Build history of the part. All positions in model axes, mm. Face numbers are marked on the shaded views. Coordinates: 2 decimals unless noted, no trailing zeros. Order: outer loops, then holes, each group sorted by start corner. A loop starts at its lowest first (then second) coordinate and runs counter-clockwise, first axis right, second up. Notation, with made-up numbers: (-8, 87) - (26, 87) arc R31 ccw to (26, 112) - close; hole circle Ø1 at (32, -15). An arc over 180 degrees is marked (long way). Write each question's results on one line, items separated by ' | '.
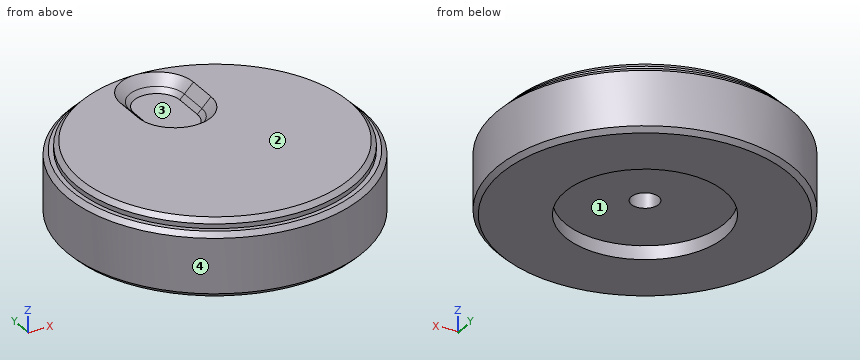
from build123d import *

# Parameters (mm, degrees)
CROQUIS1_R              = 32.5
CROQUIS1_R_2            = 3
SALIENTE_EXTRUIR1_DEPTH = 14
CROQUIS2_R              = 17.5
CORTAR_EXTRUIR1_DEPTH   = 3
CROQUIS3_R              = 30.5
SALIENTE_EXTRUIR2_DEPTH = 2
CHAFL_N1_SIZE           = 1
CORTAR_EXTRUIR2_DEPTH   = 3
CHAFL_N2_SIZE           = 2
SALIENTE_EXTRUIR3_START = 1
SALIENTE_EXTRUIR3_DEPTH = 1
CHAFL_N3_SIZE           = 1


with BuildPart() as part:
    # Croquis1 → Saliente-Extruir1 (new body)
    with BuildSketch(Plane.XY):
        Circle(CROQUIS1_R)
        Circle(CROQUIS1_R_2, mode=Mode.SUBTRACT)
    extrude(amount=SALIENTE_EXTRUIR1_DEPTH)

    # Croquis2 → Cortar-Extruir1 (cut)
    with BuildSketch(Plane(origin=(0, 0, 0), x_dir=(-1, 0, 0), z_dir=(0, 0, -1))):
        Circle(CROQUIS2_R)
    extrude(amount=-CORTAR_EXTRUIR1_DEPTH, mode=Mode.SUBTRACT)

    # Croquis3 → Saliente-Extruir2 (add)
    with BuildSketch(Plane.XY.offset(14)):
        Circle(CROQUIS3_R)
    extrude(amount=SALIENTE_EXTRUIR2_DEPTH)

    # Chaflán1
    chafl_n1_edges = [part.edges().sort_by_distance(p)[0] for p in [
        (-30.5, 0, 16),
        (-32.5, 0, 0),
        (-32.5, 0, 14),
    ]]
    chamfer(chafl_n1_edges, length=CHAFL_N1_SIZE)

    # Croquis4 → Cortar-Extruir2 (cut)
    with BuildSketch(Plane.XY.offset(16)):
        with BuildLine():
            Line((6, 21.5), (6, 15))
            ThreePointArc((6, 15), (0, 9), (-6, 15))
            Line((-6, 15), (-6, 21.5))
            ThreePointArc((-6, 21.5), (0, 27.5), (6, 21.5))
        make_face()
    extrude(amount=-CORTAR_EXTRUIR2_DEPTH, mode=Mode.SUBTRACT)

    # Chaflán2
    chafl_n2_edges = [part.edges().sort_by_distance(p)[0] for p in [
        (0, 27.5, 16),
        (-6, 18.25, 16),
        (0, 9, 16),
        (6, 18.25, 16),
    ]]
    chamfer(chafl_n2_edges, length=CHAFL_N2_SIZE - 0.0001)  # a hair under: the kernel refuses the full size

    # Croquis5 → Saliente-Extruir3 (add)
    with BuildSketch(Plane.XY.offset(13).offset(SALIENTE_EXTRUIR3_START)):
        with BuildLine():
            Line((-6, 21.5), (-6, 15))
            ThreePointArc((-6, 15), (0, 9), (6, 15))
            Line((6, 15), (6, 21.5))
            ThreePointArc((6, 21.5), (0, 27.5), (-6, 21.5))
        make_face()
        with BuildLine():
            Line((5, 15), (5, 21.5))
            ThreePointArc((5, 21.5), (0, 26.5), (-5, 21.5))
            Line((-5, 21.5), (-5, 15))
            ThreePointArc((-5, 15), (0, 10), (5, 15))
        make_face(mode=Mode.SUBTRACT)
    extrude(amount=-SALIENTE_EXTRUIR3_DEPTH)

    # Chaflán3
    chafl_n3_edges = [part.edges().sort_by_distance(p)[0] for p in [
        (5, 18.25, 14),
        (0, 26.5, 14),
        (0, 10, 14),
        (-5, 18.25, 14),
    ]]
    chamfer(chafl_n3_edges, length=CHAFL_N3_SIZE - 0.0001)  # a hair under: the kernel refuses the full size


solid = part.part
1. Band-saw the part on B-B on z = 11. Give the cut face in (x, y), then the cut area to 3 significant figures.
Solved:
outline: circle Ø65 at (0, 0); hole circle Ø6 at (0, 0) | area: 3,290 mm2
2. Probe line 1 (Y direction, x = 0, z = 6); line 2 (Y direction, x = 0, z = 1.4); line 3 (Y direction, x = 1, z = 13.25). List the from-to ranges inside material, lowest first.
Solved:
line 1: y = -32.5 to -3, 3 to 32.5 | line 2: y = -32.5 to -17.5, 17.5 to 32.5 | line 3: y = -32.23 to -2.83, 2.83 to 9.85, 26.65 to 32.23
3. Two-plate mould, pull along X, no slides. Class the marked faces 1, 2, 3 and 4: +X half, -X half, draft (parallel to the pull), parting line (faces both ways), or undercut.
Solved:
face 1: undercut | face 2: draft | face 3: undercut | face 4: parting line
4. Drop flat-ended pins along their axis: pin 1 Ø9.5 at (x, y) = (2, 16.5) entering from +Z; pin 2 Ø8 at (y, z) = (6, 7.5) entering from -X; pin 3 Ø5 at (x, y) = (0.5, 18) entering from +Z. Give the stop position or say it passes through.
Solved:
pin 1: stops at z = 14.75 | pin 2: stops at x = -32.44 | pin 3: stops at z = 13
5. Band-saw the part on A-A on y = 0. Give the cut face in (x, z).
Solved:
outline: (-32.5, 1) - (-31.5, 0) - (-17.5, 0) - (-17.5, 3) - (-3, 3) - (-3, 14) - (3, 14) - (3, 3) - (17.5, 3) - (17.5, 0) - (31.5, 0) - (32.5, 1) - (32.5, 13) - (31.5, 14) - (30.5, 14) - (30.5, 15) - (29.5, 16) - (-29.5, 16) - (-30.5, 15) - (-30.5, 14) - (-31.5, 14) - (-32.5, 13) - close
